```python
from build123d import *

# Parameters (mm, degrees)
SKETCH1_R                       = 23.114
SKETCH1_R_2                     = 9.652
BOSS_EXTRUDE1_DEPTH             = 5.08
SKETCH2_R                       = 19.939
BOSS_EXTRUDE2_DEPTH             = 101.6
BOSS_EXTRUDE2_DIRECTION_2_REACH = 35.081


with BuildPart() as part:
    # Sketch1 → Boss-Extrude1 (new body)
    with BuildSketch(Plane(origin=(0, 0, 0), x_dir=(1, 0, 0), z_dir=(0, 1, 0))):
        with Locations(Location((0, 0, 0), (0, 0, 270))):
            Circle(SKETCH1_R)
        with Locations(Location((0, 0, 0), (0, 0, 270))):
            Circle(SKETCH1_R_2, mode=Mode.SUBTRACT)
    extrude(amount=BOSS_EXTRUDE1_DEPTH)

    # Sketch2 → Boss-Extrude2 (add)
    with BuildSketch(Plane(origin=(0, 5.08, 0), x_dir=(1, 0, 0), z_dir=(0, 1, 0))):
        with BuildLine():
            Line((-14.224, 18.219078462), (-14.224, 42.164))
            Line((-14.224, 42.164), (-9.652, 42.164))
            Line((-9.652, 42.164), (-9.652, 23.114))
            Line((-9.652, 23.114), (9.652, 23.114))
            Line((9.652, 23.114), (9.652, 42.164))
            Line((9.652, 42.164), (14.224, 42.164))
            Line((14.224, 42.164), (14.224, 18.219078462))
            ThreePointArc((14.224, 18.219078462), (0, -23.114), (-14.224, 18.219078462))
        make_face()
        with Locations(Location((0, 0, 0), (0, 0, 270))):
            Circle(SKETCH2_R, mode=Mode.SUBTRACT)
    extrude(amount=BOSS_EXTRUDE2_DEPTH)

    # Boss-Extrude2 direction 2: up to this face of the body (flat: up to its plane)
    boss_extrude2_direction_2_end = Plane(part.part.faces().sort_by_distance((0, 0, -22.460237354))[0])
    # Sketch2 → Boss-Extrude2 direction 2 (add, up to the picked face)
    with BuildSketch(Plane(origin=(0, 5.08, 0), x_dir=(1, 0, 0), z_dir=(0, 1, 0)), mode=Mode.PRIVATE) as boss_extrude2_direction_2_sk1:
        with BuildLine():
            Line((-14.224, 18.219078462), (-14.224, 42.164))
            Line((-14.224, 42.164), (-9.652, 42.164))
            Line((-9.652, 42.164), (-9.652, 23.114))
            Line((-9.652, 23.114), (9.652, 23.114))
            Line((9.652, 23.114), (9.652, 42.164))
            Line((9.652, 42.164), (14.224, 42.164))
            Line((14.224, 42.164), (14.224, 18.219078462))
            ThreePointArc((14.224, 18.219078462), (0, -23.114), (-14.224, 18.219078462))
        make_face()
        with Locations(Location((0, 0, 0), (0, 0, 270))):
            Circle(SKETCH2_R, mode=Mode.SUBTRACT)
    boss_extrude2_direction_2_tool1 = split(extrude(boss_extrude2_direction_2_sk1.sketch, amount=-BOSS_EXTRUDE2_DIRECTION_2_REACH, mode=Mode.PRIVATE), bisect_by=boss_extrude2_direction_2_end, keep=Keep.BOTH, mode=Mode.PRIVATE)
    add(boss_extrude2_direction_2_tool1.solids().sort_by(Axis((-13.42411, 5.08, -30.191539), (0, -1, 0)))[0])


solid = part.part
```
Could you check a few things on this model? Use its own coordinates, in mm. A direction names the side the tool comes from. Round coordinates to 2 decimals unless told otherwise and drop trailing zeros. Loops run counter-clockwise (first coordinate to the right, second up) from the corner with the lowest first, then second, coordinate; pieces in that order, holes last. Notation, with made-up numbers: (15, -23.5) - (43, -23.5) arc R3 cw to (43, -19.5) - close; hole circle Ø2 at (61.25, -30). An arc over 180 degrees is marked (long way). Use CSV: the item, a comma, the result in double quotes.
Item 1: I need wall thicknesses on L1, parallel to X at y = 18, z = -35.5; L2, parallel to X at y = 2.25, z = 0; L3, parallel to Z at x = -21, y = 31.5. Which ranges of each line are inside material? Lowest first, please. Write a range as [from, to].
Here are the results:
L1,"x = [-14.22, -9.65], [9.65, 14.22]"
L2,"x = [-23.11, -9.65], [9.65, 23.11]"
L3,"z = [-9.66, 9.66]"
Item 2: Will these pins go through, and if not, where does the flat tip stop? pin 1 (8 mm diameter, centred on y = 76.5, z = -34, fed in from +X); pin 2 (11.5 mm diameter, centred on x = 0, z = 0, fed in from -Y); pin 3 (6 mm diameter, centred on x = -3, z = -7, fed in from +Y); pin 4 (5.5 mm diameter, centred on y = 74, z = -33.5, fed in from -X).
Here are the results:
pin 1,"stops at x = 14.22"
pin 2,"passes through"
pin 3,"stops at y = 5.08"
pin 4,"stops at x = -14.22"
Item 3: If we section it at A-A on z = 0: List the corners of the cut face in (x, y) for me.
Here are the results:
outline,"(-23.11, 0) - (-9.65, 0) - (-9.65, 5.08) - (-19.94, 5.08) - (-19.94, 106.68) - (-23.11, 106.68) - close; (9.65, 0) - (23.11, 0) - (23.11, 106.68) - (19.94, 106.68) - (19.94, 5.08) - (9.65, 5.08) - close"
Item 4: If we section it at C-C on x = 0: List the corners of the cut face in (y, z) for me, then the cut area to 3 significant figures.
Here are the results:
outline,"(0, -23.11) - (106.68, -23.11) - (106.68, -19.94) - (5.08, -19.94) - (5.08, -9.65) - (0, -9.65) - close; (0, 9.65) - (5.08, 9.65) - (5.08, 19.94) - (106.68, 19.94) - (106.68, 23.11) - (0, 23.11) - close"
area,"782 mm²"
Item 5: If we section it at B-B on y = 68: List the corners of the cut face in (x, z) for me.
Here are the results:
outline,"(-14.22, -42.16) - (-9.65, -42.16) - (-9.65, -23.11) - (9.65, -23.11) - (9.65, -42.16) - (14.22, -42.16) - (14.22, -18.22) arc R23.11 ccw (long way) to (-14.22, -18.22) - close; hole circle Ø39.88 at (0, 0)"
Item 6: If we section it at D-D on z = -33: List the corners of the cut face in (x, y) for me.
Here are the results:
outline,"(-14.22, 0) - (-9.65, 0) - (-9.65, 106.68) - (-14.22, 106.68) - close; (9.65, 0) - (14.22, 0) - (14.22, 106.68) - (9.65, 106.68) - close"
Item 7: For faces 1 (the flat face through (-9, 5.08, -5)), 2 (the flat face through (0, 54, -23.114)), 3 (the flat face through (14.224, 53, -30)), which set-ups out of +Z, -Z, +X, -X, +Y, -Y let a thin tool reach every point of the face, with its end or its side?
Here are the results:
face 1,"+Y"
face 2,"-Z, +Y, -Y"
face 3,"-Z, +X, +Y, -Y"
Item 8: If we mould it in two halves opening along X, with no side actions, what happens to faces 4 (the flat face through (-14.224, 54, -30)), 5 (the flat face through (9.652, 53, -33)), 6 (the flat face through (0, 0, -10))? For each: pulls with the +X half, pulls with the -X half, needs draft (parallel to the pull), parting line crosses it, or undercut.
Here are the results:
face 4,"pulls with the -X half"
face 5,"undercut"
face 6,"needs draft"
